from build123d import *

# Parameters (mm, degrees)
SKETCH1_W             = 32
SKETCH1_H             = 32
BOSS_EXTRUDE1_DEPTH   = 5
F_5_0MM_DOWEL_HOLE1_D = 5
F_2_0MM_DOWEL_HOLE1_D = 2
SKETCH11_W            = 32
SKETCH11_H            = 5
BOSS_EXTRUDE3_DEPTH   = 19
F_6_0MM_DOWEL_HOLE1_D = 6
SKETCH14_W            = 32
SKETCH14_H            = 5
CUT_EXTRUDE1_DEPTH    = 6
FILLET3_R             = 3


with BuildPart() as part:
    # Sketch1 → Boss-Extrude1 (new body)
    with BuildSketch(Plane.XY):
        Rectangle(SKETCH1_W, SKETCH1_H)
    extrude(amount=BOSS_EXTRUDE1_DEPTH)

    # Ø5.0mm Dowel Hole1 (through all)
    with Locations(Plane.XY.offset(5)):
        with Locations((-9, 0), (9, 0)):
            Hole(F_5_0MM_DOWEL_HOLE1_D / 2)

    # Ø2.0mm Dowel Hole1 (through all)
    with Locations(Plane.XY.offset(5)):
        with Locations((-10.5, 6.5), (10.5, 6.5), (10.5, -6.5), (-10.5, -6.5)):
            Hole(F_2_0MM_DOWEL_HOLE1_D / 2)

    # Sketch11 → Boss-Extrude3 (add)
    with BuildSketch(Plane.XY.offset(5)):
        with Locations((0, -13.5)):
            Rectangle(SKETCH11_W, SKETCH11_H)
    extrude(amount=BOSS_EXTRUDE3_DEPTH)

    # Ø6.0mm Dowel Hole1 (through all)
    with Locations(Plane(origin=(0, -11, 0), x_dir=(1, 0, 0), z_dir=(0, 1, 0))):
        with Locations((0, -15)):
            Hole(F_6_0MM_DOWEL_HOLE1_D / 2)

    # Sketch14 → Cut-Extrude1 (cut)
    with BuildSketch(Plane(origin=(0, 16, 0), x_dir=(1, 0, 0), z_dir=(0, 1, 0))):
        with Locations((0, -2.5)):
            Rectangle(SKETCH14_W, SKETCH14_H)
    extrude(amount=-CUT_EXTRUDE1_DEPTH, mode=Mode.SUBTRACT)

    # Fillet3
    fillet3_edges = [part.edges().sort_by_distance(p)[0] for p in [
        (0, -11, 5),
        (-16, -13.5, 24),
        (16, -13.5, 24),
        (16, 10, 2.5),
        (-16, 10, 2.5),
    ]]
    fillet(fillet3_edges, radius=FILLET3_R)


solid = part.part
Can you work these out from the model? Positions are in its coordinate system, mm. A direction names the side the tool comes from. Give positions to 0.01 mm unless a question says otherwise; leave off trailing zeros. Loops run counter-clockwise (first coordinate to the right, second up) from the corner with the lowest first, then second, coordinate; pieces in that order, holes last. Notation, with made-up numbers: (47.5, 61.5) - (63.5, 61.5) arc R22 ccw to (63.5, 98.5) - close; hole circle Ø10 at (-0.5, 36.5). An arc over 180 degrees is marked (long way). One line per item, written item: value.
(1) If we section it at C-C, the plane x = -10.5: List the corners of the cut face in (y, z) for me, plus the area to 3 significant figures.
Verdict:
outline: (-16, 0) - (-7.5, 0) - (-7.5, 5) - (-8, 5) arc R3 cw to (-11, 8) - (-11, 24) - (-16, 24) - close; (-5.5, 0) - (-2, 0) - (-2, 5) - (-5.5, 5) - close; (2, 0) - (5.5, 0) - (5.5, 5) - (2, 5) - close; (7.5, 0) - (10, 0) - (10, 5) - (7.5, 5) - close
area: 187 mm^2
(2) If we section it at D-D, the plane y = 0: List the corners of the cut face in (x, z) for me.
Verdict:
outline: (-16, 0) - (-11.5, 0) - (-11.5, 5) - (-16, 5) - close; (-6.5, 0) - (6.5, 0) - (6.5, 5) - (-6.5, 5) - close; (11.5, 0) - (16, 0) - (16, 5) - (11.5, 5) - close
(3) I need wall thicknesses on line 1 along Z through (x, y) = (0, -14.25); line 2 along Y through (x, z) = (10.5, 3.5); line 3 along Y through (x, z) = (-9, 1.4). Which ranges of each line are inside material? Lowest first, please.
Verdict:
line 1: 0 to 12, 18 to 24
line 2: -16 to -7.5, -5.5 to -2, 2 to 5.5, 7.5 to 10
line 3: -16 to -2.5, 2.5 to 10
(4) If we mould it in two halves opening along Z, with no side actions, what happens to faces 3 (the face through (0, -13, 24)), 4 (the face through (-9.763, -5.824, 2.465)), 5 (the face through (0.65, -13.53, 17.93))? For each: released by +Z, released by -Z, zero draft, split by the parting line, or undercut.
Verdict:
face 3: released by +Z
face 4: zero draft
face 5: undercut
(5) If we section it at A-A, the plane x = -7: List the corners of the cut face in (y, z) for me.
Verdict:
outline: (-16, 0) - (-1.5, 0) - (-1.5, 5) - (-8, 5) arc R3 cw to (-11, 8) - (-11, 24) - (-16, 24) - close; (1.5, 0) - (10, 0) - (10, 5) - (1.5, 5) - close
(6) If we section it at B-B, the plane y = -14: List the corners of the cut face in (x, z) for me, plus the area to 3 significant figures.
Verdict:
outline: (-16, 0) - (16, 0) - (16, 21) arc R3 ccw to (13, 24) - (-13, 24) arc R3 ccw to (-16, 21) - close; hole circle Ø6 at (0, 15)
area: 736 mm^2
(7) On a 3-axis mill with a long thin cutter (end or side, diameter ignored), from which of +Z, -Z, +X, -X, +Y, -Y can I reach the whole of each face in a straight line? I mean faces 1 (the face through (0, -11, 19)), 2 (the face through (-16, -10, 3)). Say none if no direction works.
Verdict:
face 1: +Z, +X, -X, +Y
face 2: +Z, -Z, -X, +Y, -Y
(8) I'm going to push flat-ended pins straight in: pin 1 (9.5 mm diameter, centred on x = 0, z = 15, fed in from +Y); pin 2 (8 mm diameter, centred on x = 1, y = -2, fed in from +Z). Where does each tip first touch, or does it pass through?
Verdict:
pin 1: y = -11
pin 2: z = 5
